CAD build for the part. Positions are in the model's coordinates, mm. Face numbers are marked on the shaded views. A direction names the side the tool comes from. Give positions to 0.01 mm unless a question says otherwise; leave off trailing zeros. Order: outer loops, then holes, each group sorted by start corner. A loop starts at its lowest first (then second) coordinate and runs counter-clockwise, first axis right, second up.
Item 1: Flat gauge pins, fed straight in: P1, Ø1, axis at y = -7.5, z = -4, coming from the -X side; P2, Ø3.5, axis at x = 4.51, y = 12.19, coming from the +Z side; P3, Ø1, axis at x = -3.5, z = -4, coming from the +Y side. Where does each tip first touch, or does it go through?
Item 2: Two-plate mould, pull along Y, no slides. Class the marked faces 4, 5 and 6: released by +Y, released by -Y, zero draft, split by the parting line, or undercut.
Item 3: Which spindle directions (+Z, -Z, +X, -X, +Y, -Y) get a long thin tool onto all of the face, cutting with end or side? Do the marked faces 1, 2 and 3. Say none if no direction does.
Item 4: Band-saw the part on D-D on x = -4.5. Give the cut face in (y, z).
Item 5: Band-saw the part on B-B on z = -1. Give the cut face in (x, y), plus the area to 3 significant figures.
Item 6: Wall check: L1, parallel to X at y = -13, z = -4; L2, parallel to X at y = 11, z = -4.5; L3, parallel to X at y = -0.5, z = 0.75. Give the ranges that are in metal, low to high.
Item 7: Band-saw the part on C-C on x = -7. Give the cut face in (y, z), plus the area to 3 significant figures.
Item 8: Band-saw the part on A-A on y = 0. Give the cut face in (x, z), plus the area to 3 significant figures.
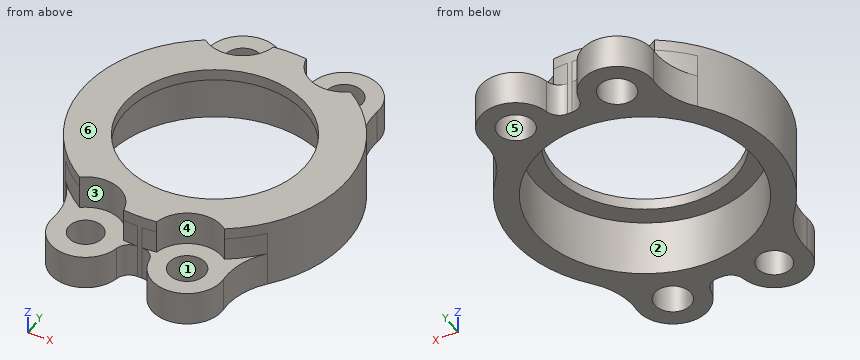
```python
from build123d import *
from build123d.topology import SkipClean

# Parameters (mm, degrees)
SKETCH1_R           = 1.6
SKETCH1_R_2         = 9.7
SKETCH1_R_3         = 1.5
BOSS_EXTRUDE1_DEPTH = 5
BOSS_EXTRUDE2_START = 1
SKETCH1_3_R         = 8
BOSS_EXTRUDE2_DEPTH = 1
FILLET1_R           = 6
FILLET5_R           = 1.25
CUT_EXTRUDE1_START  = 1
CUT_EXTRUDE1_DEPTH  = 3


with BuildPart() as part:
    # Sketch1 → Boss-Extrude1 (new body)
    with BuildSketch(Plane.XY):
        with BuildLine():
            ThreePointArc((6.440028886, -9.768112814), (11.7, 0), (6.440028886, 9.768112814))
            ThreePointArc((6.440028886, 9.768112814), (5.583978873, 15.100635084), (1.464516076, 11.607979698))
            ThreePointArc((1.464516076, 11.607979698), (0, 11.7), (-1.464516076, 11.607979698))
            ThreePointArc((-1.464516076, 11.607979698), (-5.583978873, 15.100635084), (-6.440028886, 9.768112814))
            ThreePointArc((-6.440028886, 9.768112814), (-11.7, 0), (-6.440028886, -9.768112814))
            ThreePointArc((-6.440028886, -9.768112814), (-5.583978873, -15.100635084), (-1.464516076, -11.607979698))
            ThreePointArc((-1.464516076, -11.607979698), (0, -11.7), (1.464516076, -11.607979698))
            ThreePointArc((1.464516076, -11.607979698), (5.583978873, -15.100635084), (6.440028886, -9.768112814))
        make_face()
        with Locations((-4.508802817, 12.193059385)):
            Circle(SKETCH1_R, mode=Mode.SUBTRACT)
        with Locations((4.508802817, 12.193059385)):
            Circle(SKETCH1_R, mode=Mode.SUBTRACT)
        Circle(SKETCH1_R_2, mode=Mode.SUBTRACT)
        with Locations((4.508802817, -12.193059385)):
            Circle(SKETCH1_R, mode=Mode.SUBTRACT)
        with Locations((-4.508802817, -12.193059385)):
            Circle(SKETCH1_R_3, mode=Mode.SUBTRACT)
    extrude(amount=-BOSS_EXTRUDE1_DEPTH)

    # Sketch1<3> → Boss-Extrude2 (add)
    with BuildSketch(Plane.XY.offset(BOSS_EXTRUDE2_START)):
        with BuildLine():
            ThreePointArc((6.440028886, -9.768112814), (11.7, 0), (6.440028886, 9.768112814))
            ThreePointArc((6.440028886, 9.768112814), (3.433626761, 9.285483685), (1.464516076, 11.607979698))
            ThreePointArc((1.464516076, 11.607979698), (0, 11.7), (-1.464516076, 11.607979698))
            ThreePointArc((-1.464516076, 11.607979698), (-3.433626761, 9.285483685), (-6.440028886, 9.768112814))
            ThreePointArc((-6.440028886, 9.768112814), (-11.7, 0), (-6.440028886, -9.768112814))
            ThreePointArc((-6.440028886, -9.768112814), (-3.433626761, -9.285483685), (-1.464516076, -11.607979698))
            ThreePointArc((-1.464516076, -11.607979698), (0, -11.7), (1.464516076, -11.607979698))
            ThreePointArc((1.464516076, -11.607979698), (3.433626761, -9.285483685), (6.440028886, -9.768112814))
        make_face()
        Circle(SKETCH1_3_R, mode=Mode.SUBTRACT)
    extrude(amount=-BOSS_EXTRUDE2_DEPTH)

    # Fillet1
    fillet1_edges = [part.edges().sort_by_distance(p)[0] for p in [
        (-6.440028886, -9.768112814, -2.5),
        (-6.440028886, 9.768112814, -2.5),
        (6.440028886, 9.768112814, -2.5),
        (6.440028886, -9.768112814, -2.5),
    ]]
    fillet(fillet1_edges, radius=FILLET1_R)

    # Fillet5
    fillet5_edges = [part.edges().sort_by_distance(p)[0] for p in [
        (-1.464516076, 11.607979698, -2.5),
        (1.464516076, 11.607979698, -2.5),
        (1.464516076, -11.607979698, -2.5),
        (-1.464516076, -11.607979698, -2.5),
    ]]
    fillet(fillet5_edges, radius=FILLET5_R)

    # Sketch2 → Cut-Extrude1 (cut)
    with SkipClean():  # the faces are left unmerged after this step: merging them gives an invalid solid
        with BuildSketch(Plane.XY.offset(CUT_EXTRUDE1_START)):
            with BuildLine():
                ThreePointArc((-1.464516076, -11.607979698), (-3.433626761, -9.285483685), (-6.440028886, -9.768112814))
                ThreePointArc((-6.440028886, -9.768112814), (-7.78749678, -8.731832219), (-8.970582034, -7.511235449))
                ThreePointArc((-8.970582034, -7.511235449), (-7.843991966, -9.57352888), (-7.59588423, -11.910343363))
                ThreePointArc((-7.59588423, -11.910343363), (-4.919534521, -15.265729147), (-1.455850964, -12.73109747))
                ThreePointArc((-1.455850964, -12.73109747), (-1.020006813, -11.983589345), (-0.203121026, -11.698236698))
                ThreePointArc((-0.203121026, -11.698236698), (-0.835038896, -11.67016324), (-1.464516076, -11.607979698))
            make_face()
            with BuildLine():
                ThreePointArc((6.440028886, -9.768112814), (3.433626761, -9.285483685), (1.464516076, -11.607979698))
                ThreePointArc((1.464516076, -11.607979698), (0.835038896, -11.67016324), (0.203121026, -11.698236698))
                ThreePointArc((0.203121026, -11.698236698), (1.020006813, -11.983589345), (1.455850964, -12.73109747))
                ThreePointArc((1.455850964, -12.73109747), (4.919534521, -15.265729147), (7.59588423, -11.910343363))
                ThreePointArc((7.59588423, -11.910343363), (7.843991966, -9.57352888), (8.970582034, -7.511235449))
                ThreePointArc((8.970582034, -7.511235449), (7.78749678, -8.731832219), (6.440028886, -9.768112814))
            make_face()
            with BuildLine():
                ThreePointArc((-6.440028886, 9.768112814), (-3.433626761, 9.285483685), (-1.464516076, 11.607979698))
                ThreePointArc((-1.464516076, 11.607979698), (-0.835038896, 11.67016324), (-0.203121026, 11.698236698))
                ThreePointArc((-0.203121026, 11.698236698), (-1.020006813, 11.983589345), (-1.455850964, 12.73109747))
                ThreePointArc((-1.455850964, 12.73109747), (-4.919534521, 15.265729147), (-7.59588423, 11.910343363))
                ThreePointArc((-7.59588423, 11.910343363), (-7.843991966, 9.57352888), (-8.970582034, 7.511235449))
                ThreePointArc((-8.970582034, 7.511235449), (-7.78749678, 8.731832219), (-6.440028886, 9.768112814))
            make_face()
            with BuildLine():
                ThreePointArc((1.464516076, 11.607979698), (3.433626761, 9.285483685), (6.440028886, 9.768112814))
                ThreePointArc((6.440028886, 9.768112814), (7.78749678, 8.731832219), (8.970582034, 7.511235449))
                ThreePointArc((8.970582034, 7.511235449), (7.843991966, 9.57352888), (7.59588423, 11.910343363))
                ThreePointArc((7.59588423, 11.910343363), (4.919534521, 15.265729147), (1.455850964, 12.73109747))
                ThreePointArc((1.455850964, 12.73109747), (1.020006813, 11.983589345), (0.203121026, 11.698236698))
                ThreePointArc((0.203121026, 11.698236698), (0.835038896, 11.67016324), (1.464516076, 11.607979698))
            make_face()
        extrude(amount=-CUT_EXTRUDE1_DEPTH, mode=Mode.SUBTRACT)


solid = part.part
```
The answers:
1. P1: stops at x = -9.37
1. P2: stops at z = -2
1. P3: stops at y = 15.25
2. face 4: released by -Y
2. face 5: undercut
2. face 6: zero draft
3. face 1: +Z, -Z
3. face 2: -Z
3. face 3: +Z, -Y
4. outline: (-15.29, -5) - (-13.69, -5) - (-13.69, -2) - (-15.29, -2) - close; (-10.69, -5) - (-8.59, -5) - (-8.59, 0) - (-6.61, 0) - (-6.61, 1) - (-9.09, 1) - (-9.09, -2) - (-10.69, -2) - close; (6.61, 0) - (8.59, 0) - (8.59, -5) - (10.59, -5) - (10.59, -2) - (9.09, -2) - (9.09, 1) - (6.61, 1) - close; (13.79, -5) - (15.29, -5) - (15.29, -2) - (13.79, -2) - close
5. outline: (-6.44, -9.77) arc R3.1 cw to (-1.46, -11.61) arc R11.7 ccw to (1.46, -11.61) arc R3.1 cw to (6.44, -9.77) arc R11.7 ccw to (6.44, 9.77) arc R3.1 cw to (1.46, 11.61) arc R11.7 ccw to (-1.46, 11.61) arc R3.1 cw to (-6.44, 9.77) arc R11.7 ccw to start; hole circle Ø19.4 at (0, 0)
5. area: 108 mm2
6. L1: x = -7.5 to -5.77, -3.24 to -1.52, 1.52 to 3.13, 5.89 to 7.5
6. L2: x = -7.58 to -5.57, -3.44 to 3.44, 5.57 to 7.58
6. L3: x = -11.69 to -7.98, 7.98 to 11.69
7. outline: (-14.04, -5) - (-6.71, -5) - (-6.71, 0) - (-3.87, 0) - (-3.87, 1) - (-9.37, 1) - (-9.37, -2) - (-14.04, -2) - close; (3.87, 0) - (6.71, 0) - (6.71, -5) - (14.04, -5) - (14.04, -2) - (9.37, -2) - (9.37, 1) - (3.87, 1) - close
7. area: 65.6 mm2
8. outline: (-11.7, -5) - (-9.7, -5) - (-9.7, 0) - (-8, 0) - (-8, 1) - (-11.7, 1) - close; (8, 0) - (9.7, 0) - (9.7, -5) - (11.7, -5) - (11.7, 1) - (8, 1) - close
8. area: 27.4 mm2
